Here's how the part is built. I have some questions about the finished solid (model axes, mm). Coordinates: 2 decimals unless noted, no trailing zeros. Order: outer loops, then holes, each group sorted by start corner. A loop starts at its lowest first (then second) coordinate and runs counter-clockwise, first axis right, second up. Notation, with made-up numbers: M 34.5,-23 L 68.5,-23 A24 cw 68.5,6 Z; hole C 45.25,73 d5. An arc over 180 degrees is marked long. One line per question, with ' | ' between items. Start each with the question number.
```python
from build123d import *

# Parameters (mm, degrees)
F0_R     = 6.35
F1_DEPTH = 63.5
F3_R     = 6.35
F4_DEPTH = 6.35
F5_D     = 6.35
F5_DEPTH = 63.5
F5_TIP   = 1.9077324654
F6_R     = 1.7663179958
F6_R_2   = 1.7000002335
F6_R_3   = 1.8274467347
F6_R_4   = 2.00164436
F7_DEPTH = 5.08
F8_SIZE  = 1.524


with BuildPart() as f1:
    # F0 (on Top) → F1 (new body)
    with BuildSketch(Plane.XY):
        with Locations((-23.0151098222, -49.1751506925)):
            Circle(F0_R)
    extrude(amount=F1_DEPTH)

    # F3 (on face) → F4 (join)
    with BuildSketch(Plane.XY.offset(63.5)):
        with Locations((-23.0151098222, -49.1751506925)):
            Circle(F3_R)
    extrude(amount=F4_DEPTH)

    # F5 (one way)
    with BuildSketch(Plane.XY.offset(63.5)):
        with Locations((-23.0151098222, -49.1751506925)):
            Circle(F5_D / 2)
    extrude(amount=-F5_DEPTH, mode=Mode.SUBTRACT)
    with Locations(Plane.XY.offset(63.5)):
        with Locations((-23.0151098222, -49.1751506925)):
            with Locations((0, 0, -(F5_DEPTH + F5_TIP / 2))):  # 118° drill point
                Cone(0, F5_D / 2, F5_TIP, mode=Mode.SUBTRACT)

    # F6 (on face) → F7 (join)
    with BuildSketch(Plane.XY.offset(69.85)):
        with Locations((-24.4727507234, -45.552957803)):
            Circle(F6_R)
        with Locations((-20.0130287558, -47.4362969398)):
            Circle(F6_R_2)
        with Locations((-21.5983316302, -52.6342540979)):
            Circle(F6_R_3)
        with Locations((-27.2251553833, -49.9814078212)):
            Circle(F6_R_4)
    extrude(amount=F7_DEPTH)

    # F8
    f8_edges = [f1.edges().sort_by_distance(p)[0] for p in [
        (-29.2268, -49.981408, 74.93),
        (-26.239069, -45.552958, 74.93),
        (-21.713029, -47.436297, 74.93),
        (-23.425778, -52.634254, 74.93),
    ]]
    chamfer(f8_edges, length=F8_SIZE)


solid = f1.part
```
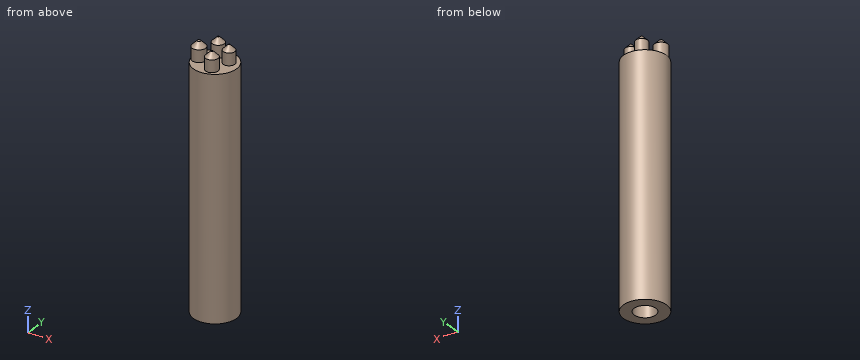
1. I need wall thicknesses on line 1 (Z direction, x = -24.75, y = -53.75); line 2 (Z direction, x = -25.25, y = -48.5); line 3 (Y direction, x = -20.25, z = 57.5). Which ranges of each line are inside material? Lowest first, please.
2. Imagine slicing it at A-A (z = 56.5). List the corners of the cut face in (x, y) for me (3 decimals).
3. Will these pins go through, and if not, where does the flat tip stop? pin 1 (1.5 mm diameter, centred on y = -53, z = 23, fed in from +X); pin 2 (1 mm diameter, centred on y = -48.5, z = 65, fed in from -X); pin 3 (6 mm diameter, centred on y = -53, z = 14.5, fed in from +X).
Entries:
1) line 1: 0 to 69.85 | line 2: 63.5 to 69.85 | line 3: -54.89 to -50.74, -47.61 to -43.46
2) outline: C -23.015,-49.175 d12.7; hole C -23.015,-49.175 d6.35
3) pin 1: x = -17.46 | pin 2: x = -29.36 | pin 3: x = -16.72
